```python
from build123d import *

# Parameters (mm, degrees)
F1_DEPTH  = 1
F2_W      = 77.1699883044
F2_H      = 14.0396282077
F2_H_2    = 14.4938565791
F2_H_3    = 13.3186802268
F3_DEPTH  = 25.4
F5_DEPTH  = 25.4
F7_DEPTH  = 25.4
F9_DEPTH  = 25.4
F12_DEPTH = 25.4
F14_DEPTH = 25.4


with BuildPart() as f1:
    # F0 (on Front) → F1 (new body)
    with BuildSketch(Plane.XZ):
        Polygon((95.7224294543, -60.3764280677), (95.7224294543, 60.3764280677), (-95.7224294543, 60.3764280677), (-95.7224294543, 44.296272099), (-18.052238971, 44.296272099), (-18.052238971, -45.8132624626), (-95.7224294543, -45.8132624626), (-95.7224294543, -60.3764280677), align=None)
    extrude(amount=F1_DEPTH)

    # F2 (on face) → F3 (cut)
    with BuildSketch(Plane.XZ.offset(1)):
        with Locations((28.3021917567, 44.296272099)):
            Rectangle(F2_W, F2_H)
        with Locations((28.3021917567, 0)):
            Rectangle(F2_W, F2_H_2)
        with Locations((28.3021917567, -45.0484715402)):
            Rectangle(F2_W, F2_H_3)
    extrude(amount=-F3_DEPTH, mode=Mode.SUBTRACT)

    # F4 (on face) → F5 (cut)
    with BuildSketch(Plane.XZ.offset(1)):
        Polygon((84.501597172, -18.5892991722), (69.1369175911, -18.5892991722), (69.1369175911, -60.3764280677), (95.7224294543, -60.3764280677), (95.7224294543, -7.0018698461), align=None)
        Polygon((69.1369175911, 60.3764280677), (69.1369175911, 19.0698392689), (84.4565480947, 19.0698392689), (95.7224294543, 7.2190617211), (95.7224294543, 60.3764280677), align=None)
    extrude(amount=-F5_DEPTH, mode=Mode.SUBTRACT)

    # F6 (on face) → F7 (cut)
    with BuildSketch(Plane.XZ.offset(1)):
        Polygon((-95.7224294543, 60.3764280677), (-95.7224294543, 52.3363500834), (-88.4090960026, 60.3764280677), align=None)
        Polygon((-88.4090960026, 44.296272099), (-95.7224294543, 52.3363500834), (-95.7224294543, 44.296272099), align=None)
    extrude(amount=-F7_DEPTH, mode=Mode.SUBTRACT)

    # F8 (on face) → F9 (cut)
    with BuildSketch(Plane.XZ.offset(1)):
        Polygon((-95.7224294543, -45.8132624626), (-95.7224294543, -53.0948452652), (-87.6560211182, -45.8132624626), align=None)
        Polygon((-87.6560211182, -60.3764280677), (-95.7224294543, -53.0948452652), (-95.7224294543, -60.3764280677), align=None)
    extrude(amount=-F9_DEPTH, mode=Mode.SUBTRACT)

    # F11 (on face) → F12 (cut)
    with BuildSketch(Plane.XZ.offset(1)):
        Polygon((-85.7021808624, 44.3187952042), (-95.5954936845, 52.1968003835), (-88.429583239, 44.3187952042), align=None)
        Polygon((-88.4090960026, 60.3764280677), (-94.2494603717, 53.9556918474), (-87.5151380897, 59.4371178139), (-88.2796930664, 60.3764280677), align=None)
    extrude(amount=-F12_DEPTH, mode=Mode.SUBTRACT)

    # F13 (on face) → F14 (cut)
    with BuildSketch(Plane.XZ.offset(1)):
        Polygon((-93.3957355305, 54.8942534959), (-95.6290065626, 52.4390566453), (-86.1386760037, 60.3764280677), (-88.4090960026, 60.3764280677), align=None)
        Polygon((-86.1098706364, 44.296272099), (-95.6111442944, 52.2140062342), (-88.4090960026, 44.296272099), align=None)
    extrude(amount=-F14_DEPTH, mode=Mode.SUBTRACT)


solid = f1.part
```
Can you work these out from the model? Positions are in its coordinate system, mm. Coordinates: 2 decimals unless noted, no trailing zeros. Write each loop counter-clockwise with the first axis right and the second up, starting at its lowest first coordinate (ties: lowest second). Pieces come first, ordered by that corner, then holes. Notation, with made-up numbers: M 8,-12.75 L 26,-12.75 A16 cw 26,14.25 Z; hole C 64.25,-2.5 d1. An arc over 180 degrees is marked long. Answer as CSV lines item,"result".
Item 1: We'd pull the mould along Z, two halves only. Please class faces 1 (the flat face through (-90.524, -0.507, 48.159)), 2 (the flat face through (20, 0, 14)), 3 (the flat face through (90.01, -0.51, 13.23)), 4 (the flat face through (-91.75, -0.51, -49.51)): +Z half, -Z half, draft (parallel to the pull), parting line (faces both ways), or undercut.
Geometry results:
face 1,"undercut"
face 2,"draft"
face 3,"+Z half"
face 4,"undercut"
Item 2: I'm going to push flat-ended pins straight in: P1, Ø0.5, axis at y = -0.5, z = 42.5, coming from the +X side; P2, Ø0.5, axis at y = -0.5, z = 13, coming from the -X side. Where does each tip first touch, or does it pass through?
Geometry results:
P1,"stops at x = 69.14"
P2,"stops at x = -18.05"
Item 3: Imagine slicing it at B-B on z = 41. List the corners of the cut face in (x, y) for me.
Geometry results:
outline,"M -18.05,-1 L -10.28,-1 L -10.28,0 L -18.05,0 Z; M 66.89,-1 L 69.14,-1 L 69.14,0 L 66.89,0 Z"
Item 4: Imagine slicing it at C-C on y = -0.55. State how many separate pieces and enclosed holes the cut face has, plus the area to 3 significant figures.
Geometry results:
separate pieces,"1"
enclosed holes,"3"
area,"10,400 mm2"
Item 5: Imagine slicing it at D-D on z = -29.5. List the corners of the cut face in (x, y) for me, plus the area to 3 significant figures.
Geometry results:
outline,"M -18.05,-1 L 69.14,-1 L 69.14,0 L -18.05,0 Z"
area,"87.2 mm2"
Item 6: Please list where these lines run through material, in increasing order: line 1 along Z through (x, y) = (49.5, -0.3); line 2 along Z through (x, y) = (-56, -0.7); line 3 along X through (y, z) = (-0.5, 47).
Geometry results:
line 1,"z = -60.38 to -51.71, -38.39 to -7.25, 7.25 to 37.28, 51.32 to 60.38"
line 2,"z = -60.38 to -45.81, 44.3 to 60.38"
line 3,"x = -89.07 to -10.28, 66.89 to 69.14"
Item 7: Imagine slicing it at A-A on x = -36. List the corners of the cut face in (y, z) for me.
Geometry results:
outline,"M -1,-60.38 L 0,-60.38 L 0,-45.81 L -1,-45.81 Z; M -1,44.3 L 0,44.3 L 0,60.38 L -1,60.38 Z"
